Read the model definition and answer for the solid it produces. Units are mm, in the model's axes. Give positions to 0.01 mm unless a question says otherwise; leave off trailing zeros. Write each loop counter-clockwise with the first axis right and the second up, starting at its lowest first coordinate (ties: lowest second). Pieces come first, ordered by that corner, then holes. Notation, with made-up numbers: (-7, 70.25) -> (35, 70.25) arc R15 cw to (35, 84.25) -> close; hole circle Ø10 at (4.5, 10). An arc over 180 degrees is marked (long way). Answer as CSV lines item,"result". Start each with the question number.
1. The part is cut by section C-C, the plane z = 0.75. Determine the outline of the cut face in (x, y), and give its area (3 significant figures).
2. The part is cut by section D-D, the plane x = -19.5. Determine the outline of the cut face in (y, z), and give its area (3 significant figures).
3. Given pin 1 (5 mm diameter, centred on x = -5.5, y = -34, fed in from -Z); pin 2 (0.6 mm diameter, centred on x = 35.5, z = 1.5, fed in from -Y); pin 3 (0.6 mm diameter, centred on x = 0, z = 0.5, fed in from -Y); pin 4 (0.6 mm diameter, centred on x = 36, z = 1, fed in from +Y), each flat-ended and moving along its own axis, determine where each tip first touches the part or whether it passes through.
4. The part is cut by section B-B, the plane y = -27. Determine the outline of the cut face in (x, z).
5. The part is cut by section A-A, the plane x = 0. Determine the outline of the cut face in (y, z), and give its area (3 significant figures).
6. Find the intervals of material crossed by line 1 (Y direction, x = 0, z = 1.5); line 2 (X direction, y = -21, z = 0.65); line 3 (Y direction, x = 15.5, z = 0.85), in increasing order.
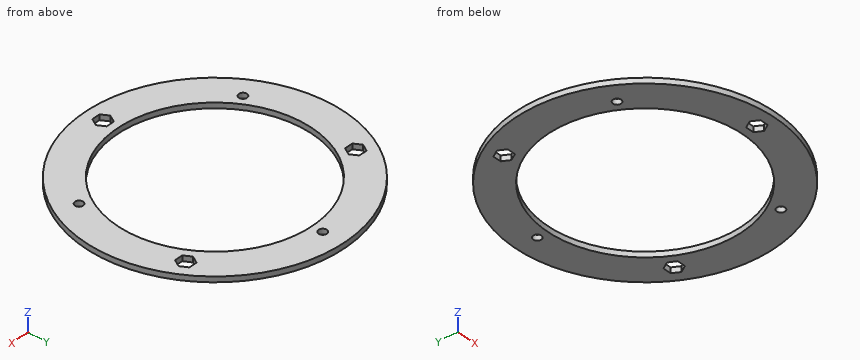
from build123d import *

# Parameters (mm, degrees)
F0_R     = 48
F0_R_2   = 1.5
F0_R_3   = 36
F1_DEPTH = 2


with BuildPart() as f1:
    # F0 (on Top) → F1 (new body)
    with BuildSketch(Plane.XY):
        Circle(F0_R)
        Polygon((-3.059956, -41.5), (-1.529978, -38.85), (1.529978, -38.85), (3.059956, -41.5), (1.529978, -44.15), (-1.529978, -44.15), align=None, mode=Mode.SUBTRACT)
        with Locations((-34.641016, -20)):
            Circle(F0_R_2, mode=Mode.SUBTRACT)
        with Locations((34.641016, -20)):
            Circle(F0_R_2, mode=Mode.SUBTRACT)
        Polygon((-32.880098, 20.75), (-34.410076, 18.1), (-37.470032, 18.1), (-39.000011, 20.75), (-37.470032, 23.4), (-34.410076, 23.4), align=None, mode=Mode.SUBTRACT)
        Circle(F0_R_3, mode=Mode.SUBTRACT)
        Polygon((34.410076, 18.1), (32.880098, 20.75), (34.410076, 23.4), (37.470032, 23.4), (39.000011, 20.75), (37.470032, 18.1), align=None, mode=Mode.SUBTRACT)
        with Locations((0, 40)):
            Circle(F0_R_2, mode=Mode.SUBTRACT)
    extrude(amount=F1_DEPTH)


solid = f1.part
Results found:
1,outline,"circle Ø96 at (0, 0); hole (-39, 20.75) -> (-37.47, 18.1) -> (-34.41, 18.1) -> (-32.88, 20.75) -> (-34.41, 23.4) -> (-37.47, 23.4) -> close; hole circle Ø3 at (-34.64, -20); hole circle Ø72 at (0, 0); hole (-3.06, -41.5) -> (-1.53, -44.15) -> (1.53, -44.15) -> (3.06, -41.5) -> (1.53, -38.85) -> (-1.53, -38.85) -> close; hole circle Ø3 at (0, 40); hole (32.88, 20.75) -> (34.41, 18.1) -> (37.47, 18.1) -> (39, 20.75) -> (37.47, 23.4) -> (34.41, 23.4) -> close; hole circle Ø3 at (34.64, -20)"
1,area,"3,070 mm²"
2,outline,"(-43.86, 0) -> (-30.26, 0) -> (-30.26, 2) -> (-43.86, 2) -> close; (30.26, 0) -> (43.86, 0) -> (43.86, 2) -> (30.26, 2) -> close"
2,area,"54.4 mm²"
3,pin 1,"stops at z = 0"
3,pin 2,"stops at y = -32.63"
3,pin 3,"stops at y = -48"
3,pin 4,"stops at y = 32.09"
4,outline,"(-39.69, 0) -> (-23.81, 0) -> (-23.81, 2) -> (-39.69, 2) -> close; (23.81, 0) -> (39.69, 0) -> (39.69, 2) -> (23.81, 2) -> close"
5,outline,"(-48, 0) -> (-44.15, 0) -> (-44.15, 2) -> (-48, 2) -> close; (-38.85, 0) -> (-36, 0) -> (-36, 2) -> (-38.85, 2) -> close; (36, 0) -> (38.5, 0) -> (38.5, 2) -> (36, 2) -> close; (41.5, 0) -> (48, 0) -> (48, 2) -> (41.5, 2) -> close"
5,area,"31.4 mm²"
6,line 1,"y = -48 to -44.15, -38.85 to -36, 36 to 38.5, 41.5 to 48"
6,line 2,"x = -43.16 to -35.76, -33.52 to -29.24, 29.24 to 33.52, 35.76 to 43.16"
6,line 3,"y = -45.43 to -32.49, 32.49 to 45.43"
